Input: part model. Units: mm. Frame: model coordinates. Coordinates: 2 decimals unless noted, no trailing zeros. Write each loop counter-clockwise with the first axis right and the second up, starting at its lowest first coordinate (ties: lowest second). Pieces come first, ordered by that corner, then holes. Notation, with made-up numbers: (58, -30.75) - (96, -30.75) arc R20 cw to (96, -0.75) - close; hole circle Ø3 at (-34, 12). An arc over 180 degrees is marked (long way). One line per question, with ' | ' between items. Start each with the question number.
1) Section query B-B on y = -40. Return loops of the section in (x, z), and give its area (3 significant figures).
2) Section query C-C on z = 74. Return loops of the section in (x, y), and give its area (3 significant figures).
3) First-contact query: P1, Ø6, axis at x = -14.5, y = -22.5, coming from the +Z side; P2, Ø20, axis at x = 0, z = 64.26, coming from the -Y side. Flat tips, straight axial feed; report the tip coordinate or a pass-through.
4) Section query A-A on x = 0. Return loops of the section in (y, z), and give its area (3 significant figures).
5) Section query D-D on x = 18.5. Return loops of the section in (y, z), and give its area (3 significant figures).
6) Draft query along Z for faces 1 (the flat face through (0, -57.404, 18)), 2 (the cylindrical face through (-2.701, -28.3, 52.093)), 3 (the cylindrical face through (0.74, -28.3, 98.06)). Return one class per face: released by +Z, released by -Z, zero draft, split by the parting line, or undercut.
7) Line query: line 1 (Z direction, x = 0, y = -24); line 2 (X direction, y = -35.5, z = 72.5); line 3 (Z direction, x = -7.5, y = -6.5). Output: solid intervals per line, ascending.
```python
from build123d import *

# Parameters (mm, degrees)
F0_R     = 12.459608
F1_DEPTH = 57.404


with BuildPart() as f1:
    # F0 (on Front) → F1 (new body)
    with BuildSketch(Plane.XZ):
        with BuildLine():
            Line((34.117013, -64.256385), (34.117013, 64.256385))
            Line((34.117013, 64.256385), (33.811439, 64.256385))
            ThreePointArc((33.811439, 64.256385), (0, 98.067824), (-33.811439, 64.256385))
            Line((-33.811439, 64.256385), (-34.117013, 64.256385))
            Line((-34.117013, 64.256385), (-34.117013, -64.256385))
            Line((-34.117013, -64.256385), (34.117013, -64.256385))
        make_face()
        with Locations((0, 64.256385)):
            Circle(F0_R, mode=Mode.SUBTRACT)
    extrude(amount=F1_DEPTH)


solid = f1.part
```
Answer key:
1) outline: (-34.12, -64.26) - (34.12, -64.26) - (34.12, 64.26) - (33.81, 64.26) arc R33.81 ccw to (-33.81, 64.26) - (-34.12, 64.26) - close; hole circle Ø24.92 at (0, 64.26) | area: 10,100 mm²
2) outline: (-32.38, -57.4) - (-7.77, -57.4) - (-7.77, 0) - (-32.38, 0) - close; (7.77, -57.4) - (32.38, -57.4) - (32.38, 0) - (7.77, 0) - close | area: 2,830 mm²
3) P1: z = 96.05 | P2: through
4) outline: (-57.4, -64.26) - (0, -64.26) - (0, 51.8) - (-57.4, 51.8) - close; (-57.4, 76.72) - (0, 76.72) - (0, 98.07) - (-57.4, 98.07) - close | area: 7,890 mm²
5) outline: (-57.4, -64.26) - (0, -64.26) - (0, 92.56) - (-57.4, 92.56) - close | area: 9,000 mm²
6) face 1: zero draft | face 2: undercut | face 3: released by +Z
7) line 1: -64.26 to 51.8, 76.72 to 98.07 | line 2: -32.79 to -9.34, 9.34 to 32.79 | line 3: -64.26 to 54.31, 74.21 to 97.23
